Input: dimensioned drawing with shaded views. Units: mm. Origin: part minimum x, y, z. A direction names the side the tool comes from. Round coordinates to 2 decimals unless told otherwise and drop trailing zeros. Write each loop counter-clockwise with the first axis right and the second up, starting at its lowest first coordinate (ties: lowest second). Pieces come first, ordered by that corner, then holes. Notation, with made-up numbers: (53, 51) -> (67, 51) arc R19 ccw to (67, 74) -> close; hole circle Ø10 at (33.5, 13). An arc over 180 degrees is marked (long way). One line per item, written item: value. Start each with the question number.
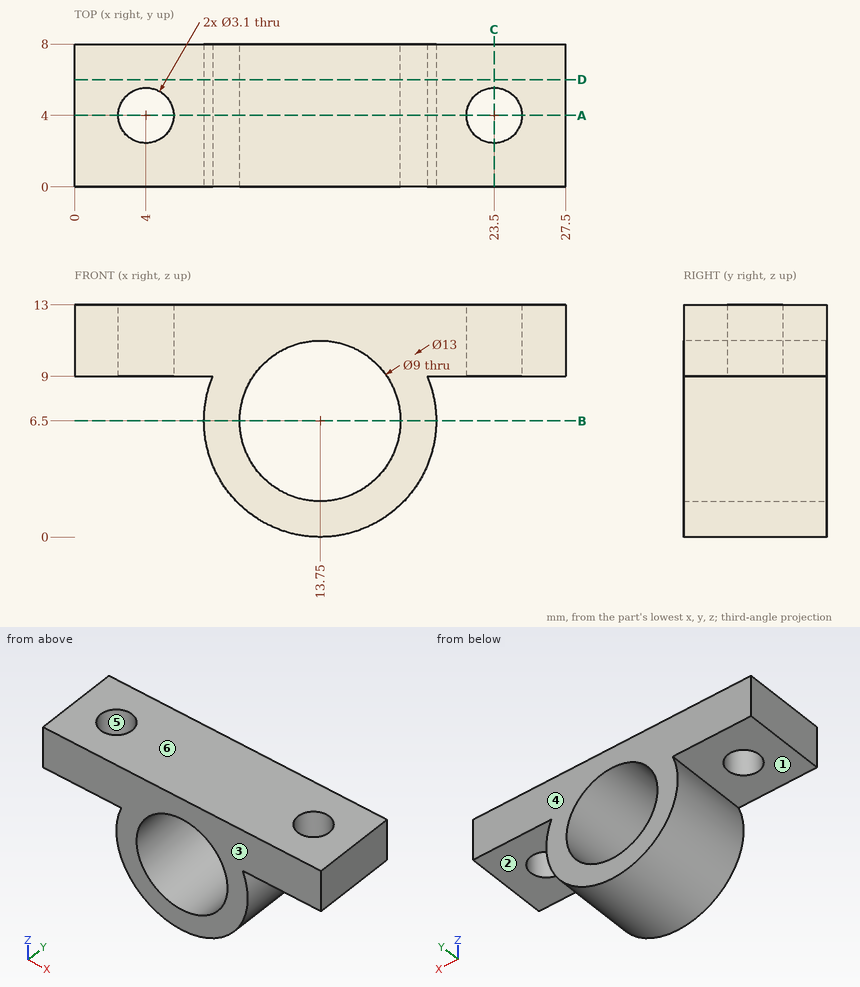
(1) Section query C-C (x = 23.5). Output: boundary loops of the cut face in (y, z).
(2) Section query A-A (y = 4). Output: boundary loops of the cut face in (x, z).
(3) Set-up query: the marked faces 1, 2 and 3. Return all of +Z, -Z, +X, -X, +Y, -Y with unobstructed straight access to the full face (end or side cutting, diameter ignored); none if empty.
(4) Line query: probe 1 along Z at (x, y) = (14, 0.5); probe 2 along X at (y, z) = (4.5, 10.5); probe 3 along X at (y, z) = (6, 6.5). Output: solid intervals per line, ascending.
(5) Pull-direction query (Y, two-part tool) for the marked faces 4, 5 and 6; classes: pulls with the +Y half, pulls with the -Y half, needs draft (parallel to the pull), parting line crosses it, or undercut.
(6) Section query B-B (z = 6.5). Output: boundary loops of the cut face in (x, y), and give its area (3 significant figures).
(7) Pin query (flat end, axial travel): pin 1 (3 mm diameter, centred on x = 24, z = 10, fed in from -Y). Return the tip coordinate at first contact, or that it passes through.
(8) Section query D-D (y = 6). Output: boundary loops of the cut face in (x, z), and give its area (3 significant figures).
Results list:
1. outline: (0, 9) -> (2.45, 9) -> (2.45, 13) -> (0, 13) -> close; (5.55, 9) -> (8, 9) -> (8, 13) -> (5.55, 13) -> close
2. outline: (0, 9) -> (2.45, 9) -> (2.45, 13) -> (0, 13) -> close; (5.55, 9) -> (7.75, 9) arc R6.5 ccw (long way) to (19.75, 9) -> (21.95, 9) -> (21.95, 13) -> (5.55, 13) -> close; (25.05, 9) -> (27.5, 9) -> (27.5, 13) -> (25.05, 13) -> close; hole circle Ø9 at (13.75, 6.5)
3. face 1: -X, +Y, -Y
3. face 2: +X, +Y, -Y
3. face 3: +Z, -Z, +X, -X, -Y
4. probe 1: z = 0 to 2.01, 10.99 to 13
4. probe 2: x = 0 to 2.53, 5.47 to 11.69, 15.81 to 22.03, 24.97 to 27.5
4. probe 3: x = 7.25 to 9.25, 18.25 to 20.25
5. face 4: pulls with the +Y half
5. face 5: undercut
5. face 6: needs draft
6. outline: (7.25, 0) -> (9.25, 0) -> (9.25, 8) -> (7.25, 8) -> close; (18.25, 0) -> (20.25, 0) -> (20.25, 8) -> (18.25, 8) -> close
6. area: 32.0 mm^2
7. pin 1: stops at y = 0
8. outline: (0, 9) -> (7.75, 9) arc R6.5 ccw (long way) to (19.75, 9) -> (27.5, 9) -> (27.5, 13) -> (0, 13) -> close; hole circle Ø9 at (13.75, 6.5)
8. area: 144 mm^2
